Source: CAD feature listing. Evaluate the final solid. Frame: model axes, mm. A direction names the side the tool comes from. Give positions to 0.01 mm unless a question says otherwise; leave off trailing zeros. Write each loop counter-clockwise with the first axis right and the second up, starting at its lowest first coordinate (ties: lowest second). Pieces come first, ordered by that corner, then holes. Notation, with made-up numbers: (-5, 25) -> (52, 25) arc R16 cw to (52, 32) -> close; hole circle Ø6 at (-8, 33.25). An arc over 180 degrees is marked (long way). Write item = value, one per line.
from build123d import *

# Parameters (mm, degrees)
F1_DEPTH = 18
F2_R     = 2.2
F2_R_2   = 1.15
F3_DEPTH = 3.001
F2_R_3   = 2.95
F4_DEPTH = 1
F5_R     = 2.2
F6_DEPTH = 3
F5_R_2   = 2.95
F7_DEPTH = 1


with BuildPart() as f1:
    # F0 (on Right) → F1 (new body)
    with BuildSketch(Plane.YZ):
        with BuildLine():
            Line((-20.2248597033, 3), (-20.2248597033, 0))
            Line((-20.2248597033, 0), (12.7751402967, 0))
            ThreePointArc((12.7751402967, 0), (13.5282296336, 1.3368087613), (12.9983799607, 2.776760336))
            Line((12.9983799607, 2.776760336), (4.9426106974, 10.8325295992))
            ThreePointArc((4.9426106974, 10.8325295992), (3.2406453095, 11.3975075099), (1.7700242043, 10.3712717737))
            Line((1.7700242043, 10.3712717737), (-1.373686309, 4.5705663947))
            ThreePointArc((-1.373686309, 4.5705663947), (-2.4763679927, 3.4223750451), (-4.0112457051, 3))
            Line((-4.0112457051, 3), (-20.2248597033, 3))
        make_face()
        with BuildLine():
            Line((4.5510043656, 6.9814952439), (8.7936450527, 2.7388545568))
            ThreePointArc((8.7936450527, 2.7388545568), (9.0865382716, 2.0317477756), (8.7936450527, 1.3246409944))
            ThreePointArc((8.7936450527, 1.3246409944), (8.0865382716, 1.0317477756), (7.3794314904, 1.3246409944))
            Line((7.3794314904, 1.3246409944), (3.1367908032, 5.5672816816))
            ThreePointArc((3.1367908032, 5.5672816816), (2.8438975844, 6.2743884627), (3.1367908032, 6.9814952439))
            ThreePointArc((3.1367908032, 6.9814952439), (3.8438975844, 7.2743884627), (4.5510043656, 6.9814952439))
        make_face(mode=Mode.SUBTRACT)
    extrude(amount=F1_DEPTH)

    # F2 (on face) → F3 (cut, through all)
    with BuildSketch(Plane.XY.offset(3)):
        with Locations((9, -11.2248597033)):
            Circle(F2_R)
        with Locations((3, -11.2248597033)):
            Circle(F2_R)
        with Locations((4.7573593129, -6.9822190162)):
            Circle(F2_R_2)
        with Locations((4.7573593129, -15.4675003905)):
            Circle(F2_R_2)
        with Locations((9, -17.2248597033)):
            Circle(F2_R)
        with Locations((13.2426406871, -15.4675003905)):
            Circle(F2_R_2)
        with Locations((15, -11.2248597033)):
            Circle(F2_R)
        with Locations((13.2426406871, -6.9822190162)):
            Circle(F2_R_2)
        with BuildLine():
            ThreePointArc((9, -20.2248597033), (2.6360389693, -17.588820734), (0, -11.2248597033))
            Line((0, -11.2248597033), (0, -20.2248597033))
            Line((0, -20.2248597033), (9, -20.2248597033))
        make_face()
        with BuildLine():
            ThreePointArc((18, -11.2248597033), (15.3639610307, -17.588820734), (9, -20.2248597033))
            Line((9, -20.2248597033), (18, -20.2248597033))
            Line((18, -20.2248597033), (18, -11.2248597033))
        make_face()
    extrude(amount=-F3_DEPTH, mode=Mode.SUBTRACT)

    # F2 (on face) → F4 (cut)
    with BuildSketch(Plane.XY.offset(3)):
        with BuildLine():
            ThreePointArc((4.9097033132, -8.9764084018), (5.5227261776, -5.1344599512), (3.2395309996, -8.284600378))
            ThreePointArc((3.2395309996, -8.284600378), (0.05, -11.2248597033), (3.2395309996, -14.1651190287))
            ThreePointArc((3.2395309996, -14.1651190287), (3.3431457505, -16.8817139528), (6.0597406747, -16.9853287037))
            ThreePointArc((6.0597406747, -16.9853287037), (9, -20.1748597033), (11.9402593253, -16.9853287037))
            ThreePointArc((11.9402593253, -16.9853287037), (14.6568542495, -16.8817139528), (14.7604690004, -14.1651190287))
            ThreePointArc((14.7604690004, -14.1651190287), (17.95, -11.2248597033), (14.7604690004, -8.284600378))
            ThreePointArc((14.7604690004, -8.284600378), (12.4772738224, -5.1344599512), (13.0902966868, -8.9764084018))
            ThreePointArc((13.0902966868, -8.9764084018), (12.05, -11.2248597033), (13.0902966868, -13.4733110049))
            ThreePointArc((13.0902966868, -13.4733110049), (11.8284271247, -14.0532868281), (11.2484513015, -15.3151563901))
            ThreePointArc((11.2484513015, -15.3151563901), (9, -14.2748597033), (6.7515486985, -15.3151563901))
            ThreePointArc((6.7515486985, -15.3151563901), (6.1715728753, -14.0532868281), (4.9097033132, -13.4733110049))
            ThreePointArc((4.9097033132, -13.4733110049), (5.95, -11.2248597033), (4.9097033132, -8.9764084018))
        make_face()
        with Locations((4.7573593129, -15.4675003905)):
            Circle(F2_R_2, mode=Mode.SUBTRACT)
        with Locations((9, -17.2248597033)):
            Circle(F2_R, mode=Mode.SUBTRACT)
        with Locations((13.2426406871, -15.4675003905)):
            Circle(F2_R_2, mode=Mode.SUBTRACT)
        with Locations((3, -11.2248597033)):
            Circle(F2_R, mode=Mode.SUBTRACT)
        with Locations((4.7573593129, -6.9822190162)):
            Circle(F2_R_2, mode=Mode.SUBTRACT)
        with Locations((15, -11.2248597033)):
            Circle(F2_R, mode=Mode.SUBTRACT)
        with Locations((13.2426406871, -6.9822190162)):
            Circle(F2_R_2, mode=Mode.SUBTRACT)
        with Locations((9, -11.2248597033)):
            Circle(F2_R_3)
        with Locations((9, -11.2248597033)):
            Circle(F2_R, mode=Mode.SUBTRACT)
    extrude(amount=-F4_DEPTH, mode=Mode.SUBTRACT)

    # F5 (on face) → F6 (cut, through all)
    with BuildSketch(Plane(origin=(0, 7.8875701483, 7.8875701483), x_dir=(-1, 0, 0), z_dir=(0, 0.7071067812, 0.7071067812))):
        with Locations((-15, -1.5314874776)):
            Circle(F5_R)
        with Locations((-9, -1.5314874776)):
            Circle(F5_R)
        with Locations((-3, -1.5314874776)):
            Circle(F5_R)
    extrude(amount=-F6_DEPTH, mode=Mode.SUBTRACT)

    # F5 (on face) → F7 (cut)
    with BuildSketch(Plane(origin=(0, 7.8875701483, 7.8875701483), x_dir=(-1, 0, 0), z_dir=(0, 0.7071067812, 0.7071067812))):
        with Locations((-15, -1.5314874776)):
            Circle(F5_R_2)
        with Locations((-15, -1.5314874776)):
            Circle(F5_R, mode=Mode.SUBTRACT)
        with Locations((-9, -1.5314874776)):
            Circle(F5_R_2)
        with Locations((-9, -1.5314874776)):
            Circle(F5_R, mode=Mode.SUBTRACT)
        with Locations((-3, -1.5314874776)):
            Circle(F5_R_2)
        with Locations((-3, -1.5314874776)):
            Circle(F5_R, mode=Mode.SUBTRACT)
    extrude(amount=-F7_DEPTH, mode=Mode.SUBTRACT)


solid = f1.part
(1) Material intervals for line 1 (X direction, y = -16, z = 0.75); line 2 (Y direction, x = 9, z = 1.75); line 3 (X direction, y = -6.5, z = 1.25), sorted ascending.
Values follow:
line_1 = 1.37 to 3.74, 5.78 to 7.17, 10.83 to 12.22, 14.26 to 16.63
line_2 = -20.22 to -19.42, -15.02 to -13.42, -9.02 to 6.95, 9.05 to 13.51
line_3 = 0 to 3.71, 5.8 to 12.2, 14.29 to 18
(2) Section query A-A (y = -6.5). Return loops of the section in (x, z).
Values follow:
outline = (0, 0) -> (3.71, 0) -> (3.71, 2) -> (2.82, 2) -> (2.82, 3) -> (0, 3) -> close; (5.8, 0) -> (12.2, 0) -> (12.2, 2) -> (11.3, 2) -> (11.3, 3) -> (6.7, 3) -> (6.7, 2) -> (5.8, 2) -> close; (14.29, 0) -> (18, 0) -> (18, 3) -> (15.18, 3) -> (15.18, 2) -> (14.29, 2) -> close
(3) Section query D-D (z = 9.5). Return loops of the section in (x, y), plus the area to 3 significant figures.
Values follow:
outline = (0, 1.3) -> (18, 1.3) -> (18, 6.28) -> (0, 6.28) -> close
area = 89.6 mm2
(4) Section query B-B (x = 10). Give the number of separate pieces and of enclosed holes in the cut face, plus the area to 3 significant figures.
Values follow:
separate_pieces = 3
enclosed_holes = 0
area = 117 mm2
(5) Access query for faces 4 (the face through (10.18, -9.37, 1.01)), 5 (the face through (6.826, -9.231, 2.507)). Directions: +Z, -Z, +X, -X, +Y, -Y. A direction counts if a zero-diameter tool reaches every point of the face in a straight line with its end or side. Return the directions, or none.
Values follow:
face_4 = +Z, -Z
face_5 = +Z
(6) First-contact query: pin 1 (9.5 mm diameter, centred on x = 15, y = -11.22, fed in from -Z); pin 2 (1 mm diameter, centred on x = 2, z = 9.5, fed in from -Y); pin 3 (1.8 mm diameter, centred on x = 10.5, y = -10.5, fed in from +Z); pin 4 (7 mm diameter, centred on x = 9, y = -11.22, fed in from +Z). Flat tips, straight axial feed; report the tip coordinate or a pass-through.
Values follow:
pin_1 = 0
pin_2 = 1.03
pin_3 = 2
pin_4 = 3
(7) Section query C-C (y = -2.5). Return loops of the section in (x, z), plus the area to 3 significant figures.
Values follow:
outline = (0, 0) -> (18, 0) -> (18, 3.41) -> (0, 3.41) -> close
area = 61.4 mm2
(8) Pull-direction query (Z, two-part tool) for faces 1 (the face through (12.547, -5.107, 2.507)), 2 (the face through (17.341, 9.891, 5.187)), 3 (the face through (8.87, 0.22, 7.51)); classes: pulls with the +Z half, pulls with the -Z half, needs draft (parallel to the pull), parting line crosses it, or undercut.
Values follow:
face_1 = needs draft
face_2 = undercut
face_3 = pulls with the +Z half
